Autodesk Inventor part; units mm, degrees
ref_plane "YZ Plane" through (0, 0, 0) normal (1, 0, 0) x (0, 1, 0)
ref_plane "XZ Plane" through (0, 0, 0) normal (0, 1, 0) x (-1, 0, 0)
ref_plane "XY Plane" through (0, 0, 0) normal (0, 0, 1) x (1, 0, 0)
sketch "Sketch1" plane through (0, 0, 0) normal (0, 0, 1) x (1, 0, 0)
  line L0 (-22, 0) -> (22, 0) construction
  circle A0 centre (-22, 0) radius 16
  circle A1 centre (22, 0) radius 16
  line L1 (43.5, -30) -> (-43.5, -30) construction
  line L2 (-43.5, -30) -> (-43.5, 30) construction
  line L3 (-43.5, 30) -> (43.5, 30) construction
  line L4 (43.5, 30) -> (43.5, -30) construction
  line L5 (43.5, -30) -> (-43.5, 30) construction
  line L6 (-43.5, -30) -> (43.5, 30) construction
  circle A2 centre (-43.5, 30) radius 4
  circle A3 centre (0, 30) radius 4
  circle A4 centre (43.5, 30) radius 4
  circle A5 centre (43.5, -30) radius 4
  circle A6 centre (-43.5, -30) radius 4
  circle A7 centre (0, -30) radius 4
  line L7 (-52.5, -37.5) -> (52.5, -37.5)
  line L8 (52.5, -37.5) -> (52.5, 37.5)
  line L9 (52.5, 37.5) -> (-52.5, 37.5)
  line L10 (-52.5, 37.5) -> (-52.5, -37.5)
  line L11 (-52.5, -37.5) -> (52.5, 37.5) construction
  line L12 (52.5, -37.5) -> (-52.5, 37.5) construction
  line L13 (-5, -17) -> (-39, -17) construction
  line L14 (-39, -17) -> (-39, 17) construction
  line L15 (-39, 17) -> (-5, 17) construction
  line L16 (-5, 17) -> (-5, -17) construction
  line L17 (-5, -17) -> (-39, 17) construction
  line L18 (-39, -17) -> (-5, 17) construction
  line L19 (39, -17) -> (5, -17) construction
  line L20 (5, -17) -> (5, 17) construction
  line L21 (5, 17) -> (39, 17) construction
  line L22 (39, 17) -> (39, -17) construction
  line L23 (39, -17) -> (5, 17) construction
  line L24 (5, -17) -> (39, 17) construction
  circle A8 centre (-39, 17) radius 3
  circle A9 centre (-39, -17) radius 3
  circle A10 centre (-5, -17) radius 3
  circle A11 centre (-5, 17) radius 3
  circle A12 centre (5, 17) radius 3
  circle A13 centre (5, -17) radius 3
  circle A14 centre (39, -17) radius 3
  circle A15 centre (39, 17) radius 3
  point P0 (0, 0)
  point P1 (0, 0)
  dimension "d0" = 60
  dimension "d1" = 87
  dimension "d2" = 44
  dimension "d3" = 32
  dimension "d4" = 8
  dimension "d5" = 105
  dimension "d6" = 75
  dimension "d10" = 34
  dimension "d11" = 6
extrude "Extrusion1" add sketch "Sketch1" along normal blind 15
fillet "Fillet1" radius 6 4 edges at (-52.5, 37.5, 7.5) (52.5, 37.5, 7.5) (52.5, -37.5, 7.5) (-52.5, -37.5, 7.5)
sketch "Sketch2" plane through (0, 0, 15) normal (0, 0, 1) x (1, 0, 0)
  circle A0 centre (22, 0) radius 16
  circle A1 centre (-22, 0) radius 16
  line L0 (37, -11) -> (7, -11)
  line L1 (7, -11) -> (7, 11)
  line L2 (7, 11) -> (37, 11)
  line L3 (37, 11) -> (37, -11)
  line L4 (37, -11) -> (7, 11) construction
  line L5 (7, -11) -> (37, 11) construction
  line L6 (-37, -11) -> (-7, -11)
  line L7 (-7, -11) -> (-7, 11)
  line L8 (-7, 11) -> (-37, 11)
  line L9 (-37, 11) -> (-37, -11)
  line L10 (-37, -11) -> (-7, 11) construction
  line L11 (-7, -11) -> (-37, 11) construction
  point P0 (0, 0)
  dimension "d12" = 22
  dimension "d13" = 30
extrude "Extrusion2" cut sketch "Sketch2" against normal through all contours L3 A0 L0 L1 L2 | A0 L2 L3 | L3 L0 A0 | A0 L1 L2 | L0 L1 A0 | L7 A1 L6 L9 L8 | A1 L8 L7 | L7 L6 A1 | A1 L9 L8 | L6 L9 A1
properties part number "cylinder frame"
Read the model definition and answer for the solid it produces. Units are mm, in the model's axes. A direction names the side the tool comes from. Give positions to 0.01 mm unless a question says otherwise; leave off trailing zeros. Order: outer loops, then holes, each group sorted by start corner. A loop starts at its lowest first (then second) coordinate and runs counter-clockwise, first axis right, second up. Notation, with made-up numbers: (20, 54.25) -> (63, 54.25) arc R7 ccw to (63, 61.25) -> close; hole circle Ø2 at (-23, -35.75). An arc over 180 degrees is marked (long way). One line per item, written item: value. Start each with the question number.
(1) A flat-ended cylindrical pin translates along its axis: P1, Ø12, axis at x = -17.5, y = 9.5, coming from the -Z side. Find the tip coordinate at first contact, or state that the pin passes through.
(2) For a pull along Y with two mould halves and no side action, classify faces 3 (the flat face through (-37, 8, 8)), 4 (the flat face through (-1, -37.5, 7)), 5 (the flat face through (-1, 1, 15)) as released by +Y, released by -Y, zero draft, split by the parting line, or undercut.
(3) The part is cut by section D-D (z = 11). State how many separate pieces and enclosed holes the cut face has, and give its area (3 significant figures).
(4) The part is cut by section A-A (x = -43.5). Determine the outline of the cut face in (y, z), and give its area (3 significant figures).
(5) Straight lines are drawn through the part: L1, parallel to Y at x = 43.5, z = 5; L2, parallel to Y at x = 39, z = 10.75; L3, parallel to X at y = -30.5, z = 2. For each, find the intervals that lie inside material, in ascending order.
(6) The part is cut by section B-B (x = 13). Determine the outline of the cut face in (y, z).
(7) A tool of negligible diameter and unlimited length cuts with its end or side. For faces 1 (the cylindrical face through (22, 16, 7)), 2 (the cylindrical face through (-50.789, -35.696, 7.605)), from which of +Z, -Z, +X, -X, +Y, -Y can it reach the whole face along a straight path? Write none if from no direction.
(8) The part is cut by section C-C (y = -27.5). Determine the outline of the cut face in (x, z), and give its area (3 significant figures).
Taken from the geometry:
1. P1: z = 0
2. face 3: undercut
2. face 4: released by -Y
2. face 5: zero draft
3. separate pieces: 1
3. enclosed holes: 16
3. area: 5,650 mm^2
4. outline: (-37.5, 0) -> (-34, 0) -> (-34, 15) -> (-37.5, 15) -> close; (-26, 0) -> (26, 0) -> (26, 15) -> (-26, 15) -> close; (34, 0) -> (37.5, 0) -> (37.5, 15) -> (34, 15) -> close
4. area: 885 mm^2
5. L1: -37.5 to -34, -26 to 26, 34 to 37.5
5. L2: -37.5 to -20, -14 to 14, 20 to 37.5
5. L3: -52.5 to -47.47, -39.53 to -3.97, 3.97 to 39.53, 47.47 to 52.5
6. outline: (-37.5, 0) -> (-13.23, 0) -> (-13.23, 15) -> (-37.5, 15) -> close; (13.23, 0) -> (37.5, 0) -> (37.5, 15) -> (13.23, 15) -> close
7. face 1: +Z, -Z
7. face 2: +Z, -Z, -X, -Y
8. outline: (-52.5, 0) -> (-46.62, 0) -> (-46.62, 15) -> (-52.5, 15) -> close; (-40.38, 0) -> (-3.12, 0) -> (-3.12, 15) -> (-40.38, 15) -> close; (3.12, 0) -> (40.38, 0) -> (40.38, 15) -> (3.12, 15) -> close; (46.62, 0) -> (52.5, 0) -> (52.5, 15) -> (46.62, 15) -> close
8. area: 1,290 mm^2
